Part model, mm, in its own coordinate system. Face numbers are marked on the shaded views. Round coordinates to 2 decimals unless told otherwise and drop trailing zeros. Write each loop counter-clockwise with the first axis right and the second up, starting at its lowest first coordinate (ties: lowest second). Pieces come first, ordered by that corner, then holes. Notation, with made-up numbers: (10.25, 6.5) -> (45.25, 6.5) arc R11 ccw to (45.25, 26.5) -> close; hole circle Ø6 at (23, 4.5). An arc over 180 degrees is marked (long way). Use CSV: the item, a comma, the result in double quotes. Start each with the question number.
(1) Drop flat-ended pins along their axis: pin 1 (8 mm diameter, centred on x = 11.5, z = -11.5, fed in from +Y); pin 2 (4 mm diameter, centred on y = 2.5, z = -18.5, fed in from +X); pin 3 (6 mm diameter, centred on x = -23, y = 7, fed in from +Z). Give the stop position or say it passes through.
(2) Two-plate mould, pull along Z, no slides. Class the marked faces 1, 2 and 3: released by +Z, released by -Z, zero draft, split by the parting line, or undercut.
(3) Saw through at A-A (y = 3). Give the cut face in (x, z), plus the area to 3 significant figures.
(4) Probe line 1 (Y direction, x = 9, z = 1); line 2 (X direction, y = 7.5, z = 17); line 3 (Z direction, x = -18, y = 13.75). List the from-to ranges inside material, lowest first. Write a range as [from, to].
(5) Saw through at B-B (y = 9.5). Give the cut face in (x, z), plus the area to 3 significant figures.
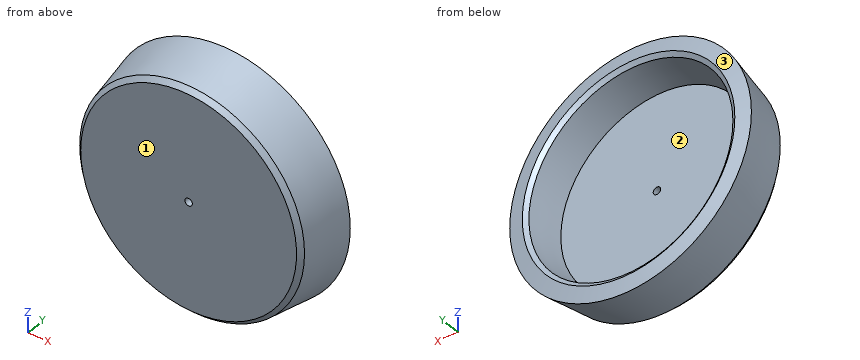
```python
from build123d import *

# Parameters (mm, degrees)
CHAMFER_1_SIZE      = 1
CHAMFER_1_SIZE2     = 1.232803052
CHAMFER_2_SIZE      = 1
SKETCH_4_R          = 1
CUT_EXTRUDE_1_DEPTH = 10


with BuildPart() as part:
    # 草图3 → 旋转1 (revolve)
    with BuildSketch(Plane.XY):
        Polygon((0, 0), (-30.195498156, 0), (-32.687308572, 14.131759112), (-27.763269807, 15), (-26, 5), (0, 5), align=None)
    revolve(axis=Axis((0, 5, 0), (0, -1, 0)))

    # 倒角1
    chamfer_1_edges = [part.edges().sort_by_distance(p)[0] for p in [
        (30.195498156, 0, 0),
    ]]
    chamfer_1_side = [part.faces().sort_by_distance(p)[0] for p in [
        (0, 0, 0),
    ]]
    chamfer(chamfer_1_edges, length=CHAMFER_1_SIZE, length2=CHAMFER_1_SIZE2, reference=chamfer_1_side[0])

    # 倒角2
    chamfer_2_edges = [part.edges().sort_by_distance(p)[0] for p in [
        (27.763269807, 15, 0),
    ]]
    chamfer(chamfer_2_edges, length=CHAMFER_2_SIZE)

    # 草图4 → 切除-拉伸1 (cut)
    with BuildSketch(Plane(origin=(0, 5, 0), x_dir=(1, 0, 0), z_dir=(0, 1, 0))):
        with Locations(Location((0, 0, 0), (0, 0, 180))):
            Circle(SKETCH_4_R)
    extrude(amount=-CUT_EXTRUDE_1_DEPTH, mode=Mode.SUBTRACT)


solid = part.part
```
Answers:
1,pin 1,"stops at y = 5"
1,pin 2,"stops at x = 25.88"
1,pin 3,"stops at z = 24.34"
2,face 1,"zero draft"
2,face 2,"undercut"
2,face 3,"split by the parting line"
3,outline,"circle Ø61.45 at (0, 0); hole circle Ø2 at (0, 0)"
3,area,"2,960 mm²"
4,line 1,"y = [0, 5]"
4,line 2,"x = [-26.54, -20.25], [20.25, 26.54]"
4,line 3,"z = [-27.2, -20.85], [20.85, 27.2]"
5,outline,"circle Ø63.74 at (0, 0); hole circle Ø53.59 at (0, 0)"
5,area,"936 mm²"
